Part model, mm, in its own coordinate system. Round coordinates to 2 decimals unless told otherwise and drop trailing zeros. Loops run counter-clockwise (first coordinate to the right, second up) from the corner with the lowest first, then second, coordinate; pieces in that order, holes last. Notation, with made-up numbers: (-34.5, 54) - (10.5, 54) arc R22 cw to (10.5, 75) - close; hole circle Ø3 at (19, 57.25). An arc over 180 degrees is marked (long way). Write each question's results on one line, items separated by ' | '. Start each with the question number.
(1) Mould opens along Y. For faces 1 (the face through (54.81, 9.04, 5.07)), 2 (the face through (94, 0, 5)), 3 (the face through (94, 50, 5)) say: released by +Y, released by -Y, zero draft, split by the parting line, or undercut.
(2) Cut at C-C, the plane x = 67. List the corners of the cut face in (y, z), then the cut area to 3 significant figures.
(3) Cut at A-A, the plane y = 10. List the corners of the cut face in (x, z), then the cut area to 3 significant figures.
(4) Cut at B-B, the plane x = 7.5. List the corners of the cut face in (y, z), then the cut area to 3 significant figures.
(5) Drill centre lines: L1, parallel to Y at x = 67.5, z = 2.25; L2, parallel to Y at x = 139, z = 9. Where is each one in solid material? Low to high.
from build123d import *

# Parameters (mm, degrees)
SKETCH_W               = 190
SKETCH_H               = 50
PAD_DEPTH              = 10
SKETCH001_R            = 2.5
HOLE_DEPTH             = 10.001
LINEARPATTERN_COUNT    = 2
LINEARPATTERN_PITCH    = 45
LINEARPATTERN001_COUNT = 2
LINEARPATTERN001_PITCH = 60
LINEARPATTERN002_COUNT = 2
LINEARPATTERN002_PITCH = 115
LINEARPATTERN003_COUNT = 2
LINEARPATTERN003_PITCH = 130
LINEARPATTERN004_COUNT = 2
LINEARPATTERN004_PITCH = 175


with BuildPart() as part:
    # Sketch → Pad (new body)
    with BuildSketch(Plane.XY):
        with Locations((95, 25)):
            Rectangle(SKETCH_W, SKETCH_H)
    extrude(amount=PAD_DEPTH)

    # Sketch001 (on Face6 of Pad) → Hole (cut, through all)
    with BuildSketch(Plane.XY.offset(10)):
        with Locations((7.5, 10)):
            Circle(SKETCH001_R)
    hole = extrude(amount=-HOLE_DEPTH, mode=Mode.SUBTRACT)

    # LinearPattern: Hole ×2
    with Locations(*[(i * LINEARPATTERN_PITCH, 0, 0) for i in range(1, LINEARPATTERN_COUNT)]):
        add(hole, mode=Mode.SUBTRACT)

    # LinearPattern001: Hole ×2
    with Locations(*[(i * LINEARPATTERN001_PITCH, 0, 0) for i in range(1, LINEARPATTERN001_COUNT)]):
        add(hole, mode=Mode.SUBTRACT)

    # LinearPattern002: Hole ×2
    with Locations(*[(i * LINEARPATTERN002_PITCH, 0, 0) for i in range(1, LINEARPATTERN002_COUNT)]):
        add(hole, mode=Mode.SUBTRACT)

    # LinearPattern003: Hole ×2
    with Locations(*[(i * LINEARPATTERN003_PITCH, 0, 0) for i in range(1, LINEARPATTERN003_COUNT)]):
        add(hole, mode=Mode.SUBTRACT)

    # LinearPattern004: Hole ×2
    with Locations(*[(i * LINEARPATTERN004_PITCH, 0, 0) for i in range(1, LINEARPATTERN004_COUNT)]):
        add(hole, mode=Mode.SUBTRACT)


solid = part.part
A:
1) face 1: undercut | face 2: released by -Y | face 3: released by +Y
2) outline: (0, 0) - (7.55, 0) - (7.55, 10) - (0, 10) - close; (12.45, 0) - (50, 0) - (50, 10) - (12.45, 10) - close | area: 451 mm2
3) outline: (0, 0) - (5, 0) - (5, 10) - (0, 10) - close; (10, 0) - (50, 0) - (50, 10) - (10, 10) - close; (55, 0) - (65, 0) - (65, 10) - (55, 10) - close; (70, 0) - (120, 0) - (120, 10) - (70, 10) - close; (125, 0) - (135, 0) - (135, 10) - (125, 10) - close; (140, 0) - (180, 0) - (180, 10) - (140, 10) - close; (185, 0) - (190, 0) - (190, 10) - (185, 10) - close | area: 1,600 mm2
4) outline: (0, 0) - (7.5, 0) - (7.5, 10) - (0, 10) - close; (12.5, 0) - (50, 0) - (50, 10) - (12.5, 10) - close | area: 450 mm2
5) L1: 0 to 7.5, 12.5 to 50 | L2: 0 to 8, 12 to 50
